```python
from build123d import *

# Parameters (mm, degrees)
SKETCH_1_R      = 50.5
SKETCH_1_R_2    = 2.6
EXTRUDE_1_DEPTH = 12
FILLET_1_R      = 10


with BuildPart() as part:
    # ｽｹｯﾁ1 → ﾎﾞｽ - 押し出し1 (new body)
    with BuildSketch(Plane(origin=(0, 0, 0), x_dir=(1, 0, 0), z_dir=(0, 1, 0))):
        with BuildLine():
            Line((-6.641105235, 63.695364835), (-10.641105235, 56.506786136))
            ThreePointArc((-10.641105235, 56.506786136), (-40.658639918, 40.658639918), (-56.506786136, 10.641105235))
            Line((-56.506786136, 10.641105235), (-63.695364835, 6.641105235))
            ThreePointArc((-63.695364835, 6.641105235), (-67.6, 0), (-63.695364835, -6.641105235))
            Line((-63.695364835, -6.641105235), (-56.506786136, -10.641105235))
            ThreePointArc((-56.506786136, -10.641105235), (-40.658639918, -40.658639918), (-10.641105235, -56.506786136))
            Line((-10.641105235, -56.506786136), (-6.641105235, -63.695364835))
            ThreePointArc((-6.641105235, -63.695364835), (0, -67.6), (6.641105235, -63.695364835))
            Line((6.641105235, -63.695364835), (10.641105235, -56.506786136))
            ThreePointArc((10.641105235, -56.506786136), (40.658639918, -40.658639918), (56.506786136, -10.641105235))
            Line((56.506786136, -10.641105235), (63.695364835, -6.641105235))
            ThreePointArc((63.695364835, -6.641105235), (67.6, 0), (63.695364835, 6.641105235))
            Line((63.695364835, 6.641105235), (56.506786136, 10.641105235))
            ThreePointArc((56.506786136, 10.641105235), (40.658639918, 40.658639918), (10.641105235, 56.506786136))
            Line((10.641105235, 56.506786136), (6.641105235, 63.695364835))
            ThreePointArc((6.641105235, 63.695364835), (0, 67.6), (-6.641105235, 63.695364835))
        make_face()
        with Locations(Location((0, 0, 0), (0, 0, 270))):
            Circle(SKETCH_1_R, mode=Mode.SUBTRACT)
        with Locations(Location((0, 60, 0), (0, 0, 270))):
            Circle(SKETCH_1_R_2, mode=Mode.SUBTRACT)
        with Locations(Location((60, 0, 0), (0, 0, 270))):
            Circle(SKETCH_1_R_2, mode=Mode.SUBTRACT)
        with Locations(Location((0, -60, 0), (0, 0, 270))):
            Circle(SKETCH_1_R_2, mode=Mode.SUBTRACT)
        with Locations(Location((-60, 0, 0), (0, 0, 270))):
            Circle(SKETCH_1_R_2, mode=Mode.SUBTRACT)
    extrude(amount=EXTRUDE_1_DEPTH)

    # ﾌｨﾚｯﾄ1
    fillet_1_edges = [part.edges().sort_by_distance(p)[0] for p in [
        (10.641105235, 6, -56.506786136),
        (56.506786136, 6, -10.641105235),
        (56.506786136, 6, 10.641105235),
        (10.641105235, 6, 56.506786136),
        (-10.641105235, 6, 56.506786136),
        (-56.506786136, 6, 10.641105235),
        (-56.506786136, 6, -10.641105235),
        (-10.641105235, 6, -56.506786136),
    ]]
    fillet(fillet_1_edges, radius=FILLET_1_R)


solid = part.part
```
Input: part model. Units: mm. Frame: model coordinates. Give positions to 0.01 mm unless a question says otherwise; leave off trailing zeros. Loops run counter-clockwise (first coordinate to the right, second up) from the corner with the lowest first, then second, coordinate; pieces in that order, holes last. Notation, with made-up numbers: (79.5, 27.5) -> (89.5, 27.5) arc R27 ccw to (89.5, 44.5) -> close; hole circle Ø4 at (19.5, 8). An arc over 180 degrees is marked (long way). Use a Markdown table: item, result.
Q1. Ray query, probe 1 along X at (y, z) = (6.25, 0); probe 2 along Z at (x, y) = (1.5, 8.5); probe 3 along Z at (x, y) = (-1, 7.25). Return the intervals inside material, ascending. Write a range as from..to.
Entries:
| item | result |
|---|---|
| probe 1 | x = -67.6..-62.6, -57.4..-50.5, 50.5..57.4, 62.6..67.6 |
| probe 2 | z = -67.45..-62.12, -57.88..-50.48, 50.48..57.88, 62.12..67.45 |
| probe 3 | z = -67.53..-62.4, -57.6..-50.49, 50.49..57.6, 62.4..67.53 |
Q2. Section query B-B, the plane z = 0. Return the cut outline in (x, y).
Entries:
| item | result |
|---|---|
| outline | (-67.6, 0) -> (-62.6, 0) -> (-62.6, 12) -> (-67.6, 12) -> close; (-57.4, 0) -> (-50.5, 0) -> (-50.5, 12) -> (-57.4, 12) -> close; (50.5, 0) -> (57.4, 0) -> (57.4, 12) -> (50.5, 12) -> close; (62.6, 0) -> (67.6, 0) -> (67.6, 12) -> (62.6, 12) -> close |
Q3. Section query A-A, the plane y = 8. State how many separate pieces and enclosed holes the cut face has, plus the area to 3 significant figures.
Entries:
| item | result |
|---|---|
| separate pieces | 1 |
| enclosed holes | 5 |
| area | 2,900 mm² |
Q4. Section query D-D, the plane z = 43. Return the cut outline in (x, y).
Entries:
| item | result |
|---|---|
| outline | (-38.17, 0) -> (-26.48, 0) -> (-26.48, 12) -> (-38.17, 12) -> close; (26.48, 0) -> (38.17, 0) -> (38.17, 12) -> (26.48, 12) -> close |
Q5. Pull-direction query (Z, two-part tool) for faces 1 (the flat face through (62.03, 5.92, 7.57)), 2 (the cylindrical face through (0.1, 5.9, 57.4)), 3 (the flat face through (7.57, 5.92, -62.03)); classes: pulls with the +Z half, pulls with the -Z half, needs draft (parallel to the pull), parting line crosses it, or undercut.
Entries:
| item | result |
|---|---|
| face 1 | pulls with the +Z half |
| face 2 | undercut |
| face 3 | pulls with the -Z half |
Q6. First-contact query: P1, Ø2, axis at x = -15, y = 1.5, coming from the -Z side; P2, Ø3, axis at y = 3, z = -30, coming from the -X side; P3, Ø1, axis at x = -30.5, y = 5, coming from the -Z side. Flat tips, straight axial feed; report the tip coordinate or a pass-through.
Entries:
| item | result |
|---|---|
| P1 | stops at z = -55.8 |
| P2 | stops at x = -49.94 |
| P3 | stops at z = -49.05 |
Q7. Section query C-C, the plane x = -22. Return the cut outline in (y, z).
Entries:
| item | result |
|---|---|
| outline | (0, -53.12) -> (12, -53.12) -> (12, -45.46) -> (0, -45.46) -> close; (0, 45.46) -> (12, 45.46) -> (12, 53.12) -> (0, 53.12) -> close |
